The drawing under review shows one solid part. Ordinate dimensions are in mm from its lowest x, y, z. A direction names the side the tool comes from. Coordinates: 2 decimals unless noted, no trailing zeros. Loops run counter-clockwise (first coordinate to the right, second up) from the corner with the lowest first, then second, coordinate; pieces in that order, holes last. Notation, with made-up numbers: (44, 20) -> (57, 20) arc R11 cw to (57, 29) -> close; hole circle Ø5 at (-3.75, 1.25). An arc over 180 degrees is marked (long way). Use a Markdown table: item, result.
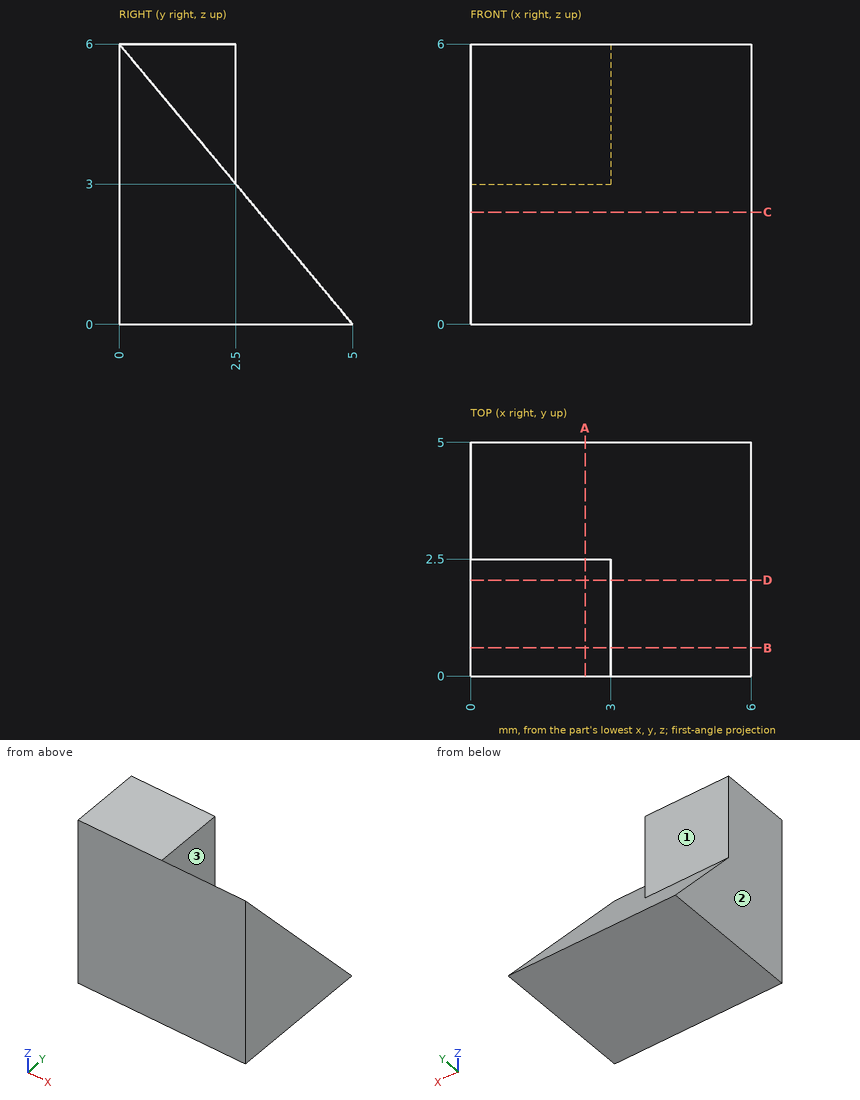
(1) Take a section at A-A on x = 2.45. Write out the cut boundary in (y, z), plus the area to 4 significant figures.
Found:
| item | result |
|---|---|
| outline | (0, 0) -> (5, 0) -> (2.5, 3) -> (2.5, 6) -> (0, 6) -> close |
| area | 18.75 mm^2 |
(2) Take a section at B-B on y = 0.6. Write out the cut boundary in (x, z).
Found:
| item | result |
|---|---|
| outline | (0, 0) -> (6, 0) -> (6, 5.28) -> (3, 5.28) -> (3, 6) -> (0, 6) -> close |
(3) For line 1 along Y through (x, z) = (2.45, 2.4); line 2 along Y through (x, z) = (1.35, 5.15), list the stretches that pass through material, from the lowest coordinate up.
Found:
| item | result |
|---|---|
| line 1 | y = 0 to 3 |
| line 2 | y = 0 to 2.5 |
(4) For pin 1 Ø3 at (x, z) = (4, 4) entering from +Y; pin 2 Ø1 at (x, y) = (5, 4) entering from -Z; pin 3 Ø3.5 at (x, z) = (2, 4) entering from +Y (3 decimals), all flat-tipped, find the tip position at first contact; note any pin that passes through.
Found:
| item | result |
|---|---|
| pin 1 | stops at y = 2.92 |
| pin 2 | stops at z = 0 |
| pin 3 | stops at y = 3.125 |
(5) For the marked faces 1, 2 and 3, list the 3-axis set-ups (+Z, -Z, +X, -X, +Y, -Y) from which the entire face can be reached by the end or side of a thin tool; tool diameter is ignored.
Found:
| item | result |
|---|---|
| face 1 | +Z, +X, -X, +Y |
| face 2 | +Z, -Z, -X, +Y, -Y |
| face 3 | +Z, +X, +Y |
(6) Take a section at D-D on y = 2.05. Write out the cut boundary in (x, z).
Found:
| item | result |
|---|---|
| outline | (0, 0) -> (6, 0) -> (6, 3.54) -> (3, 3.54) -> (3, 6) -> (0, 6) -> close |
(7) Take a section at C-C on z = 2.4. Write out the cut boundary in (x, y).
Found:
| item | result |
|---|---|
| outline | (0, 0) -> (6, 0) -> (6, 3) -> (0, 3) -> close |
